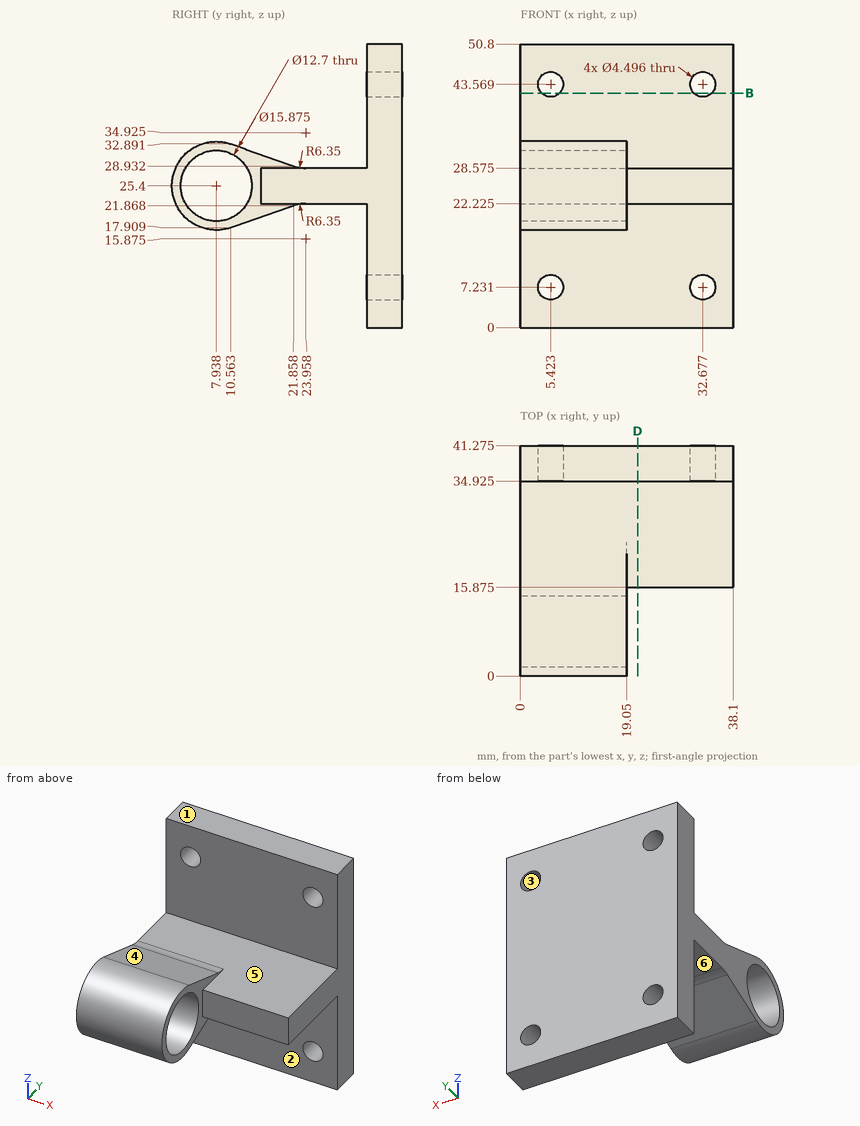
Design review of the part shown in the three views and the two pictorial views. Dimensions are in mm from the part's minimum x, y and z. A direction names the side the tool comes from. Round coordinates to 2 decimals unless told otherwise and drop trailing zeros. Write each loop counter-clockwise with the first axis right and the second up, starting at its lowest first coordinate (ties: lowest second). Pieces come first, ordered by that corner, then holes. Notation, with made-up numbers: (24.25, 8) - (29.25, 8) arc R19 ccw to (29.25, 24) - close; hole circle Ø1 at (23, -6). An arc over 180 degrees is marked (long way). Answer as CSV lines item,"result". Start each with the question number.
(1) For pin 1 (11 mm diameter, centred on x = 28, z = 45, fed in from -Y) (1 decimal); pin 2 (15 mm diameter, centred on x = 18, y = 24, fed in from -Z); pin 3 (2 mm diameter, centred on x = 10, z = 31, fed in from -Y); pin 4 (2.5 mm diameter, centred on x = 32.68, z = 7.23, fed in from -Y), all flat-tipped, find the tip position at first contact; note any pin that passes through.
(2) Mouldability with a two-part tool opening along Z and no side actions: class the marked faces 1, 2 and 3 as +Z half, -Z half, draft (parallel to the pull), parting line (faces both ways), or undercut.
(3) Add section B-B, the plane z = 42. State the section outline as (x, y) points (1 decimal).
(4) Add section D-D, the plane x = 21. State the section outline as (y, z) points (1 decimal).
(5) Machinability: for the marked faces 4, 5 and 6, which of the approach directions +Z, -Z, +X, -X, +Y, -Y give a long, thin tool a straight path to every point of the face, cutting with its end or side? Answer none if there is none.
(6) For line 1 (Y direction, x = 12, z = 25) (1 decimal); line 2 (Y direction, x = 6.5, z = 10.5) (1 decimal); line 3 (Z direction, x = 8, y = 28) (1 decimal), list the stretches that pass through material, from the lowest coordinate up.
From the geometry:
1,pin 1,"stops at y = 34.9"
1,pin 2,"stops at z = 19.99"
1,pin 3,"stops at y = 1.47"
1,pin 4,"passes through"
2,face 1,"+Z half"
2,face 2,"draft"
2,face 3,"undercut"
3,outline,"(0, 34.9) - (3.8, 34.9) - (3.8, 41.3) - (0, 41.3) - close; (7, 34.9) - (31.1, 34.9) - (31.1, 41.3) - (7, 41.3) - close; (34.3, 34.9) - (38.1, 34.9) - (38.1, 41.3) - (34.3, 41.3) - close"
4,outline,"(15.9, 22.2) - (34.9, 22.2) - (34.9, 0) - (41.3, 0) - (41.3, 50.8) - (34.9, 50.8) - (34.9, 28.6) - (15.9, 28.6) - close"
5,face 4,"+Z, +X, -X"
5,face 5,"+Z, +X"
5,face 6,"-Z, +X"
6,line 1,"y = 0 to 1.6, 14.3 to 41.3"
6,line 2,"y = 34.9 to 41.3"
6,line 3,"z = 22.2 to 28.6"
